from build123d import *

# Parameters (mm, degrees)
SKETCH1_R           = 12.5
BOSS_EXTRUDE1_DEPTH = 5
SKETCH2_R           = 7.5
BOSS_EXTRUDE2_DEPTH = 5
SKETCH3_R           = 5.5
CUT_EXTRUDE1_DEPTH  = 3.5
SKETCH6_R           = 1.75
CUT_EXTRUDE2_DEPTH  = 21


with BuildPart() as part:
    # Sketch1 → Boss-Extrude1 (new body)
    with BuildSketch(Plane(origin=(0, 0, 0), x_dir=(1, 0, 0), z_dir=(0, 1, 0))):
        Circle(SKETCH1_R)
    extrude(amount=BOSS_EXTRUDE1_DEPTH)

    # Sketch2 → Boss-Extrude2 (add)
    with BuildSketch(Plane(origin=(0, 5, 0), x_dir=(1, 0, 0), z_dir=(0, 1, 0))):
        Circle(SKETCH2_R)
    extrude(amount=BOSS_EXTRUDE2_DEPTH)

    # Mirror6: part across plane


with BuildPart() as part_1:
    add(part.part)
    add(part.part.mirror(Plane.ZX.offset(10)))

    # Sketch3 → Cut-Extrude1 (cut)
    with BuildSketch(Plane(origin=(0, 20, 0), x_dir=(1, 0, 0), z_dir=(0, 1, 0))):
        Circle(SKETCH3_R)
    extrude(amount=-CUT_EXTRUDE1_DEPTH, mode=Mode.SUBTRACT)

    # Sketch6 → Cut-Extrude2 (cut, through all)
    with BuildSketch(Plane.XZ):
        Circle(SKETCH6_R)
    extrude(amount=-CUT_EXTRUDE2_DEPTH, mode=Mode.SUBTRACT)


solid = part_1.part
Design review of the part built by this model. Coordinates are the model's own, in mm. A direction names the side the tool comes from. Round coordinates to 2 decimals unless told otherwise and drop trailing zeros. Loops run counter-clockwise (first coordinate to the right, second up) from the corner with the lowest first, then second, coordinate; pieces in that order, holes last. Notation, with made-up numbers: (-39, -19.5) - (14, -19.5) arc R32 ccw to (14, 13.5) - close; hole circle Ø3 at (-11, 2.25). An arc over 180 degrees is marked (long way). One line per question, with ' | ' between items.
1. We need section D-D, the plane z = -8.75. State the section outline as (x, y) points.
Results are:
outline: (-8.93, 0) - (8.93, 0) - (8.93, 5) - (-8.93, 5) - close; (-8.93, 15) - (8.93, 15) - (8.93, 20) - (-8.93, 20) - close
2. Clearance check with flat-ended pins moving along their axes: P1, Ø1.5, axis at x = 6.5, y = 10.5, coming from the +Z side; P2, Ø10, axis at x = 0, z = 0, coming from the +Y side; P3, Ø8, axis at y = 11.5, z = -4.5, coming from the -X side. State where each tip first meets the part, or that it passes through.
Results are:
P1: stops at z = 4.82 | P2: stops at y = 16.5 | P3: stops at x = -12.23
3. We need section B-B, the plane z = 0. State the section outline as (x, y) points, and give its area (3 significant figures).
Results are:
outline: (-12.5, 0) - (-1.75, 0) - (-1.75, 16.5) - (-5.5, 16.5) - (-5.5, 20) - (-12.5, 20) - (-12.5, 15) - (-7.5, 15) - (-7.5, 5) - (-12.5, 5) - close; (1.75, 0) - (12.5, 0) - (12.5, 5) - (7.5, 5) - (7.5, 15) - (12.5, 15) - (12.5, 20) - (5.5, 20) - (5.5, 16.5) - (1.75, 16.5) - close | area: 304 mm²
4. For faces 1 (the face through (0, 16.5, 2)), 2 (the face through (1.617, 8.134, -0.67)), 3 (the face through (0, 5, 8)), list the 3-axis set-ups (+Z, -Z, +X, -X, +Y, -Y) from which the entire face can be reached by the end or side of a thin tool; tool diameter is ignored.
Results are:
face 1: +Y | face 2: +Y, -Y | face 3: none
5. Draft analysis for pull direction Y (two halves, no side actions). For faces 4 (the face through (0, 15, 8)), 5 (the face through (0, 0, 3)), 6 (the face through (-1.19, 18.27, 5.37)), state which applies: released by +Y, released by -Y, zero draft, split by the parting line, or undercut.
Results are:
face 4: undercut | face 5: released by -Y | face 6: zero draft
6. For L1, parallel to Z at x = 0, y = 19; L2, parallel to Y at x = 11.75, z = -2.75, list the stretches that pass through material, from the lowest coordinate up. Write a range as [from, to].
Results are:
L1: z = [-12.5, -5.5], [5.5, 12.5] | L2: y = [0, 5], [15, 20]
7. We need section C-C, the plane y = 9.5. State the section outline as (x, z) points.
Results are:
outline: circle Ø15 at (0, 0); hole circle Ø3.5 at (0, 0)
8. We need section A-A, the plane x = 0. State the section outline as (y, z) points, and give its area (3 significant figures).
Results are:
outline: (0, -12.5) - (5, -12.5) - (5, -7.5) - (15, -7.5) - (15, -12.5) - (20, -12.5) - (20, -5.5) - (16.5, -5.5) - (16.5, -1.75) - (0, -1.75) - close; (0, 1.75) - (16.5, 1.75) - (16.5, 5.5) - (20, 5.5) - (20, 12.5) - (15, 12.5) - (15, 7.5) - (5, 7.5) - (5, 12.5) - (0, 12.5) - close | area: 304 mm²
